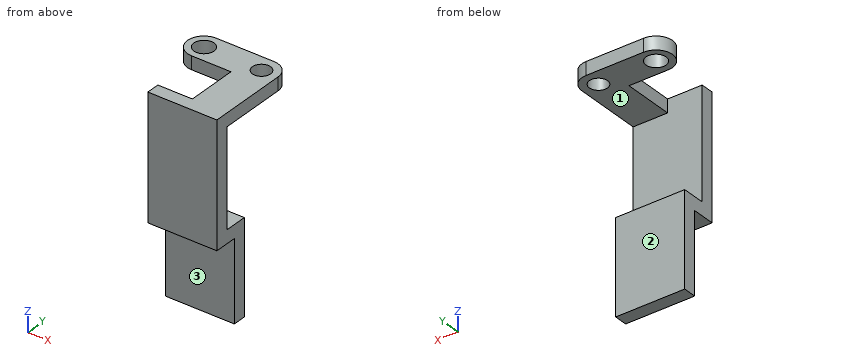
from build123d import *

# Parameters (mm, degrees)
BOSS_EXTRUDE1_DEPTH     = 42
SKETCH11_W              = 42
SKETCH11_H              = 16
BOSS_EXTRUDE2_DEPTH     = 82
BOSS_EXTRUDE4_DEPTH     = 16
CUT_EXTRUDE2_DEPTH      = 270.02044532
CUT_EXTRUDE2_DEPTH_BACK = 270.02044532
SKETCH17_R              = 11.03433716
SKETCH17_R_2            = 12.280198215


with BuildPart() as part:
    # Sketch10 → Boss-Extrude1 (new, symmetric)
    with BuildSketch(Plane(origin=(0, 0, 0), x_dir=(0, 0, -1), z_dir=(1, 0, 0))):
        Polygon((-150, 0), (0, 0), (0, 28), (98, 28), (98, 44), (-16, 44), (-16, 16), (-150, 16), align=None)
    extrude(amount=BOSS_EXTRUDE1_DEPTH, both=True)

    # Sketch11 → Boss-Extrude2 (add)
    with BuildSketch(Plane(origin=(0, 16, 0), x_dir=(1, 0, 0), z_dir=(0, 1, 0))):
        with Locations((21, -142)):
            Rectangle(SKETCH11_W, SKETCH11_H)
    extrude(amount=BOSS_EXTRUDE2_DEPTH)

    # Sketch12 → Boss-Extrude4 (add)
    with BuildSketch(Plane.XY.offset(150)):
        with BuildLine():
            Line((-48, 118), (22, 118))
            ThreePointArc((22, 118), (42, 98), (22, 78))
            Line((22, 78), (-48, 78))
            ThreePointArc((-48, 78), (-68, 98), (-48, 118))
        make_face()
    extrude(amount=-BOSS_EXTRUDE4_DEPTH)

    # Sketch17 → Cut-Extrude2 (cut, two sides: drawn at the far end of the back side and taken through both)
    with BuildSketch(Plane(origin=(0, 0, 134), x_dir=(-1, 0, 0), z_dir=(0, 0, -1)).offset(-CUT_EXTRUDE2_DEPTH_BACK)):
        with Locations(Location((-22, 98, 0), (0, 0, 90))):
            Circle(SKETCH17_R)
        with Locations(Location((48, 98, 0), (0, 0, 90))):
            Circle(SKETCH17_R_2)
    extrude(amount=CUT_EXTRUDE2_DEPTH + CUT_EXTRUDE2_DEPTH_BACK, mode=Mode.SUBTRACT)


solid = part.part
The model under review builds one solid part; all positions refer to its coordinate system, in mm. Face numbers are marked on the shaded views. A direction names the side the tool comes from. Round coordinates to 2 decimals unless told otherwise and drop trailing zeros. Loops run counter-clockwise (first coordinate to the right, second up) from the corner with the lowest first, then second, coordinate; pieces in that order, holes last. Notation, with made-up numbers: (86.5, -27) - (128.5, -27) arc R21 cw to (128.5, -23) - close; hole circle Ø10 at (7, 2). An arc over 180 degrees is marked (long way). Use CSV: the item, a comma, the result in double quotes.
(1) Take a section at D-D, the plane x = 4. Give the boundary of the cut face in (y, z), plus the area to 3 significant figures.
Working result:
outline,"(0, 0) - (28, 0) - (28, -98) - (44, -98) - (44, 16) - (16, 16) - (16, 134) - (118, 134) - (118, 150) - (0, 150) - close"
area,"6,050 mm^2"
(2) Take a section at C-C, the plane y = 106.5. Give the boundary of the cut face in (x, z), plus the area to 3 significant figures.
Working result:
outline,"(-66.1, 134) - (-56.86, 134) - (-56.86, 150) - (-66.1, 150) - close; (-39.14, 134) - (14.96, 134) - (14.96, 150) - (-39.14, 150) - close; (29.04, 134) - (40.1, 134) - (40.1, 150) - (29.04, 150) - close"
area,"1,190 mm^2"
(3) Clearance check with flat-ended pins moving along their axes: P1, Ø2, axis at x = -32.5, z = 32.5, coming from the +Y side; P2, Ø6, axis at x = -41.5, y = 93, coming from the +Z side; P3, Ø1.5, axis at x = 18.5, z = -61.5, coming from the +Y side; P4, Ø5, axis at y = 36, z = 139.5, coming from the -X side. State where each tip first meets the part, or that it passes through.
Working result:
P1,"stops at y = 16"
P2,"passes through"
P3,"stops at y = 44"
P4,"stops at x = 0"
(4) For line 1 (X direction, y = 98, z = 146.25); line 2 (Y direction, x = 22, z = 139); line 3 (X direction, y = 17, z = 12), list the stretches that pass through material, from the lowest coordinate up.
Working result:
line 1,"x = -68 to -60.28, -35.72 to 10.97, 33.03 to 42"
line 2,"y = 0 to 86.97, 109.03 to 118"
line 3,"x = -42 to 42"
(5) Take a section at A-A, the plane y = 24. Give the boundary of the cut face in (x, z), plus the area to 3 significant figures.
Working result:
outline,"(-42, 0) - (42, 0) - (42, 16) - (-42, 16) - close; (0, 134) - (42, 134) - (42, 150) - (0, 150) - close"
area,"2,020 mm^2"
(6) Machinability: for the marked faces 1, 2 and 3, which of the approach directions +Z, -Z, +X, -X, +Y, -Y give a long, thin tool a straight path to every point of the face, cutting with its end or side? Answer none if there is none.
Working result:
face 1,"+X, -X, +Y"
face 2,"-Z, +X, -X, +Y"
face 3,"-Z, +X, -X, -Y"
(7) Take a section at B-B, the plane x = -21.5. Give the boundary of the cut face in (y, z).
Working result:
outline,"(0, 0) - (28, 0) - (28, -98) - (44, -98) - (44, 16) - (16, 16) - (16, 150) - (0, 150) - close; (78, 134) - (118, 134) - (118, 150) - (78, 150) - close"
